Geometry: final body of the model. Coordinates: model frame, mm. Face numbers are marked on the shaded views. A direction names the side the tool comes from. Give positions to 0.01 mm unless a question says otherwise; leave off trailing zeros. Write each loop counter-clockwise with the first axis right and the second up, starting at its lowest first coordinate (ties: lowest second). Pieces come first, ordered by that corner, then holes. Notation, with made-up numbers: M 82.5,-19 L 88.5,-19 A7 cw 88.5,-7 Z; hole C 61,52 d10. An arc over 180 degrees is marked long. Use a Markdown table: item, result. Add a question column.
1) Line query: line 1 (X direction, y = 3.5, z = -4); line 2 (Z direction, x = 0.4, y = 0); line 3 (X direction, y = -2, z = 4). Output: solid intervals per line, ascending.
2) Draft query along X for the marked faces 5, 6, 7 and 8. Return one class per face: +X half, -X half, draft (parallel to the pull), parting line (faces both ways), or undercut.
3) Section B-B on x = 4.5. Return the cut outline in (y, z), then the cut area to 3 significant figures.
4) Set-up query: the marked faces 1, 2, 3 and 4. Return all of +Z, -Z, +X, -X, +Y, -Y with unobstructed straight access to the full face (end or side cutting, diameter ignored); none if empty.
5) Pin query (flat end, axial travel): pin 1 (1.5 mm diameter, centred on x = -8, y = -1.5, fed in from +Z); pin 2 (4 mm diameter, centred on y = -1, z = 0, fed in from -X); pin 3 (2 mm diameter, centred on x = 3, y = 0, fed in from -Z). Return the tip coordinate at first contact, or that it passes through.
6) Section A-A on x = -0.25. Return the cut outline in (y, z).
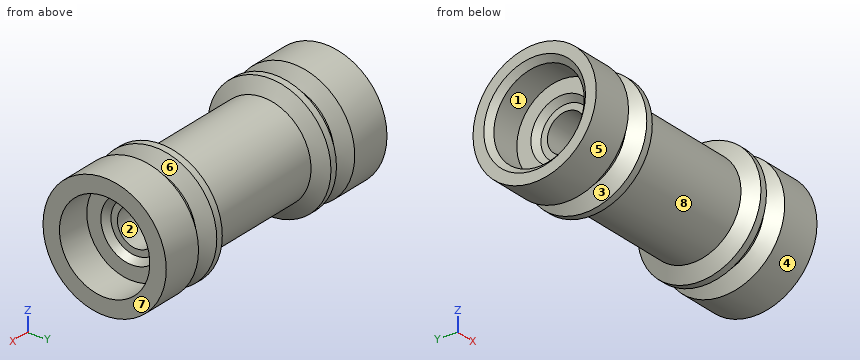
```python
from build123d import *

# Parameters (mm, degrees)
CHAMFER1_SIZE = 0.508


with BuildPart() as part:
    # Sketch2 → Revolve1 (revolve)
    with BuildSketch(Plane.XY, mode=Mode.PRIVATE) as revolve1_sk:
        Polygon((-8.988234842, 5.55625), (-12.7, 5.55625), (-12.7, 4.075), (-9.55, 4.075), (-9.55, 2.805), (-9.042, 2.297), (-9.042, 1.7145), (-2.875, 1.7145), (-2.875, 1.6), (0, 1.6), (0, 4.318), (-5.536861187, 4.318), (-6.251765158, 5.55625), (-6.886765158, 5.55625), (-7.62, 4.28625), (-8.255, 4.28625), align=None)
    revolve(revolve1_sk.sketch.rotate(Axis((-12.7, 0, 0), (1, 0, 0)), 180), axis=Axis((-12.7, 0, 0), (1, 0, 0)))

    # Mirror1: part across plane


with BuildPart() as part_1:
    add(part.part)
    add(part.part.mirror(Plane(origin=(0, 0, 0), x_dir=(0, 0, 1), z_dir=(1, 0, 0))))

    # Chamfer1
    chamfer1_edges = [part_1.edges().sort_by_distance(p)[0] for p in [
        (-12.7, 4.075, 0),
    ]]
    chamfer(chamfer1_edges, length=CHAMFER1_SIZE)


solid = part_1.part
```
Found:
| question | item | result |
|---|---|---|
| 1 | line 1 | -12.7 to -8.85, -7.03 to -6.11, 6.11 to 7.03, 8.85 to 12.7 |
| 1 | line 2 | -4.32 to -1.6, 1.6 to 4.32 |
| 1 | line 3 | -12.59 to -8.36, -7.51 to -5.63, 5.63 to 7.51, 8.36 to 12.7 |
| 2 | face 5 | draft |
| 2 | face 6 | undercut |
| 2 | face 7 | +X half |
| 2 | face 8 | undercut |
| 3 | outline | C 0,0 d8.64; hole C 0,0 d3.43 |
| 3 | area | 49.3 mm² |
| 4 | face 1 | -X |
| 4 | face 2 | +X |
| 4 | face 3 | none |
| 4 | face 4 | +X, -X |
| 5 | pin 1 | z = 4.94 |
| 5 | pin 2 | x = -9.55 |
| 5 | pin 3 | z = -4.32 |
| 6 | outline | C 0,0 d8.64; hole C 0,0 d3.2 |
